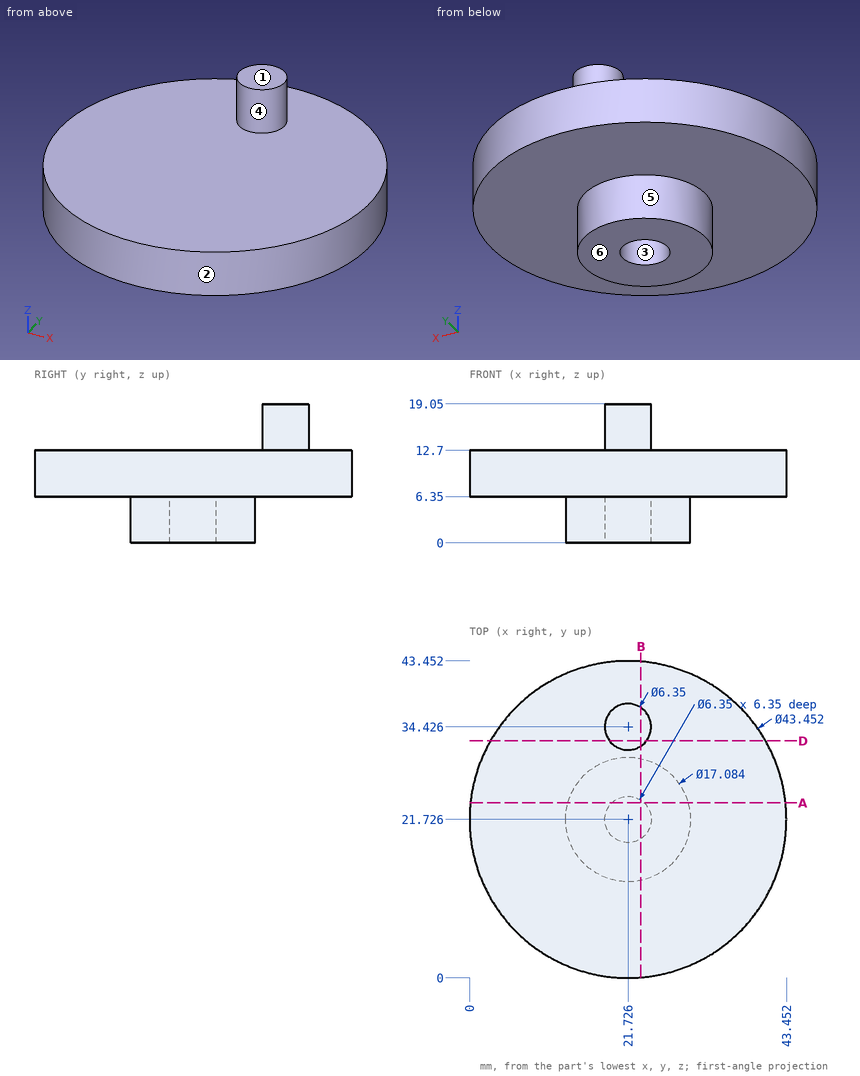
Part print with two shaded views. Sizes in mm from the minimum x, y, z corner. A direction names the side the tool comes from. Coordinates: 2 decimals unless noted, no trailing zeros. Write each loop counter-clockwise with the first axis right and the second up, starting at its lowest first coordinate (ties: lowest second). Pieces come first, ordered by that corner, then holes. Notation, with made-up numbers: (23, 46) -> (70, 46) arc R32 ccw to (70, 77) -> close; hole circle Ø3 at (25, 79.5). An arc over 180 degrees is marked (long way). Return JSON: item names as keys, results as strings. Group by question number.
Q1. Cut at A-A, the plane y = 24. Give the cut face in (x, z).
Q2. Drill centre lines: line 1 (Z direction, x = 38.5, y = 32); line 2 (Z direction, x = 14.5, y = 21); line 3 (Y direction, x = 20, z = 3). Where is each one in solid material? Low to high.
Q3. Which spindle directions (+Z, -Z, +X, -X, +Y, -Y) get a long thin tool onto all of the face, cutting with end or side? Do the marked faces 4, 5 and 6. Say none if no direction does.
Q4. Pull direction X, two halves, no side cores. Call the marked faces 1, 2 and 3: released by +X, released by -X, zero draft, split by the parting line, or undercut.
Q5. Cut at B-B, the plane x = 23.5. Give the cut face in (y, z), then the cut area to 3 significant figures.
Q6. Flat gauge pins, fed straight in: pin 1 (5 mm diameter, centred on x = 22, y = 22, fed in from -Z); pin 2 (4 mm diameter, centred on y = 30, z = 8, fed in from +X); pin 3 (1.5 mm diameter, centred on x = 9, y = 22, fed in from +Z). Where does each tip first touch, or does it go through?
Q7. Cut at D-D, the plane y = 32.5. Give the cut face in (x, z), then the cut area to 3 significant figures.
Returned:
{
 "1": {"outline": "(0.12, 6.35) -> (13.49, 6.35) -> (13.49, 0) -> (19.51, 0) -> (19.51, 6.35) -> (23.94, 6.35) -> (23.94, 0) -> (29.96, 0) -> (29.96, 6.35) -> (43.33, 6.35) -> (43.33, 12.7) -> (0.12, 12.7) -> close"},
 "2": {"line 1": "z = 6.35 to 12.7", "line 2": "z = 0 to 12.7", "line 3": "y = 13.36 to 19.06, 24.39 to 30.09"},
 "3": {"face 4": "+Z", "face 5": "-Z", "face 6": "-Z, +X, -X, +Y, -Y"},
 "4": {"face 1": "zero draft", "face 2": "split by the parting line", "face 3": "undercut"},
 "5": {"outline": "(0.07, 6.35) -> (13.37, 6.35) -> (13.37, 0) -> (19.09, 0) -> (19.09, 6.35) -> (24.36, 6.35) -> (24.36, 0) -> (30.08, 0) -> (30.08, 6.35) -> (43.38, 6.35) -> (43.38, 12.7) -> (37.06, 12.7) -> (37.06, 19.05) -> (31.79, 19.05) -> (31.79, 12.7) -> (0.07, 12.7) -> close", "area": "381 mm2"},
 "6": {"pin 1": "stops at z = 6.35", "pin 2": "stops at x = 42.53", "pin 3": "stops at z = 12.7"},
 "7": {"outline": "(2.86, 6.35) -> (40.59, 6.35) -> (40.59, 12.7) -> (24.25, 12.7) -> (24.25, 19.05) -> (19.2, 19.05) -> (19.2, 12.7) -> (2.86, 12.7) -> close", "area": "272 mm2"}
}
